```python
from build123d import *

# Parameters (mm, degrees)
SKETCH_1_W      = 350
SKETCH_1_H      = 40
SKETCH_1_R      = 2.95
EXTRUDE_1_DEPTH = 4
FILLET_1_R      = 1


with BuildPart() as part:
    # 草图1 → 凸台-拉伸1 (new body)
    with BuildSketch(Plane(origin=(0, 0, 0), x_dir=(0, 0, -1), z_dir=(1, 0, 0))):
        with Locations((175, 20)):
            Rectangle(SKETCH_1_W, SKETCH_1_H)
        with Locations((10, 30)):
            Circle(SKETCH_1_R, mode=Mode.SUBTRACT)
        with Locations((10, 10)):
            Circle(SKETCH_1_R, mode=Mode.SUBTRACT)
        with Locations(Location((340, 10, 0), (0, 0, 180))):
            Circle(SKETCH_1_R, mode=Mode.SUBTRACT)
        with Locations(Location((340, 30, 0), (0, 0, 180))):
            Circle(SKETCH_1_R, mode=Mode.SUBTRACT)
    extrude(amount=EXTRUDE_1_DEPTH)

    # 圆角1
    fillet_1_edges = [part.edges().sort_by_distance(p)[0] for p in [
        (2, 40, 0),
        (2, 40, -350),
        (2, 0, -350),
        (2, 0, 0),
    ]]
    fillet(fillet_1_edges, radius=FILLET_1_R)


solid = part.part
```
Can you work these out from the model? Positions are in its coordinate system, mm. Coordinates: 2 decimals unless noted, no trailing zeros. Order: outer loops, then holes, each group sorted by start corner. A loop starts at its lowest first (then second) coordinate and runs counter-clockwise, first axis right, second up. Notation, with made-up numbers: (-2, 20.5) -> (27, 20.5) arc R19 ccw to (27, 30.5) -> close; hole circle Ø4 at (63, 83). An arc over 180 degrees is marked (long way). Write each question's results on one line, items separated by ' | '.
Item 1: If I drill on line 1 along Y through (x, z) = (1.8, -340); line 2 along Z through (x, y) = (1.9, 31); line 3 along Z through (x, y) = (1.8, 28.5), over which ranges is the centre line in solid material (lowest first)?
Results are:
line 1: 0 to 7.05, 12.95 to 27.05, 32.95 to 40 | line 2: -350 to -342.78, -337.22 to -12.78, -7.22 to 0 | line 3: -350 to -342.54, -337.46 to -12.54, -7.46 to 0
Item 2: I want a section at A-A, the plane y = 30. Write out the boundary of the cut face in (x, z), then the cut area to 3 significant figures.
Results are:
outline: (0, -350) -> (4, -350) -> (4, -342.95) -> (0, -342.95) -> close; (0, -337.05) -> (4, -337.05) -> (4, -12.95) -> (0, -12.95) -> close; (0, -7.05) -> (4, -7.05) -> (4, 0) -> (0, 0) -> close | area: 1,350 mm²
Item 3: If we mould it in two halves opening along Y, with no side actions, what happens to faces 1 (the face through (1.972, 9.114, -337.186)), 2 (the face through (1.972, 31.994, -7.826)), 3 (the face through (0, 20, -173))? For each: +Y half, -Y half, draft (parallel to the pull), parting line (faces both ways), or undercut.
Results are:
face 1: undercut | face 2: undercut | face 3: draft
Item 4: I want a section at B-B, the plane z = -340. Write out the boundary of the cut face in (x, y), then the cut area to 3 significant figures.
Results are:
outline: (0, 0) -> (4, 0) -> (4, 7.05) -> (0, 7.05) -> close; (0, 12.95) -> (4, 12.95) -> (4, 27.05) -> (0, 27.05) -> close; (0, 32.95) -> (4, 32.95) -> (4, 40) -> (0, 40) -> close | area: 113 mm²
Item 5: I'm going to push a flat-ended pin straight in: pin 1 Ø9.5 at (y, z) = (30, -340) entering from -X. Where does the tip first touch, or does it pass through?
Results are:
pin 1: x = 0
